from build123d import *
from build123d import SkipClean  # not in build123d's __all__

# Parameters (mm, degrees)
F0_R     = 2.775
F0_R_2   = 1.275
F1_DEPTH = 2


with BuildPart() as f1:
    # F0 (on Top) → F1 (new body)
    with BuildSketch(Plane.XY):
        with BuildLine():
            Line((0, 28.575), (-45, 28.575))
            Line((-45, 28.575), (-45, -28.575))
            Line((-45, -28.575), (0, -28.575))
            Line((0, -28.575), (0, -27.8123737215))
            ThreePointArc((0, -27.8123737215), (-2.775, -25.0373737215), (0, -22.2623737215))
            Line((0, -22.2623737215), (0, 28.575))
        make_face()
        with Locations((-39, 25.075)):
            Circle(F0_R, mode=Mode.SUBTRACT)
        with BuildLine():
            Line((0, -23.7623737215), (0, -22.2623737215))
            ThreePointArc((0, -22.2623737215), (-2.775, -25.0373737215), (0, -27.8123737215))
            Line((0, -27.8123737215), (0, -26.3123737215))
            ThreePointArc((0, -26.3123737215), (-1.275, -25.0373737215), (0, -23.7623737215))
        make_face()
        with Locations((-39, 25.075)):
            Circle(F0_R)
        with Locations((-39, 25.075)):
            Circle(F0_R_2, mode=Mode.SUBTRACT)
    extrude(amount=F1_DEPTH)

    # F2: F1 across face


with BuildPart() as f1_1:
    add(f1.part, clean=False)
    with SkipClean():  # cleaning this boolean's faces spoils the solid; the shape is the same uncleaned
        add(f1.part.mirror(Plane(origin=(0, 2.4063131393, 1), x_dir=(0, 1, 0), z_dir=(1, 0, 0))), clean=False)


solid = f1_1.part
The listing builds one solid part. Answer for the finished solid, in the listing's coordinates (mm). Coordinates: 2 decimals unless noted, no trailing zeros. Write each loop counter-clockwise with the first axis right and the second up, starting at its lowest first coordinate (ties: lowest second). Pieces come first, ordered by that corner, then holes. Notation, with made-up numbers: (61, 9) - (87, 9) arc R13 cw to (87, 22) - close; hole circle Ø3 at (66, 80). An arc over 180 degrees is marked (long way). Return JSON: item names as keys, results as strings.
1. For a pull along Y with two mould halves and no side action, classify faces 1 (the face through (1, -28.575, 1)), 2 (the face through (-45, 0, 1)), 3 (the face through (0.056, -23.764, 0.986)) as +Y half, -Y half, draft (parallel to the pull), parting line (faces both ways), or undercut.
Final values:
{"face 1": "-Y half", "face 2": "draft", "face 3": "undercut"}
2. Consider line 1 along X through (y, z) = (-25, 0.35); line 2 along Y through (x, z) = (-39, 0.65) (3 decimals); line 3 along X through (y, z) = (24.5, 0.65). Determine where each line is inside the solid, lowest interval first.
Final values:
{"line 1": "-45 to -1.27, 1.27 to 45", "line 2": "-28.575 to 23.8, 26.35 to 28.575", "line 3": "-45 to -40.14, -37.86 to 37.86, 40.14 to 45"}
3. The part is cut by section B-B on y = -25. Determine the outline of the cut face in (x, z).
Final values:
{"outline": "(-45, 0) - (-1.27, 0) - (-1.27, 2) - (-45, 2) - close; (1.27, 0) - (45, 0) - (45, 2) - (1.27, 2) - close"}
4. The part is cut by section A-A on x = 0. Determine the outline of the cut face in (y, z) (3 decimals), then the cut area to 3 significant figures.
Final values:
{"outline": "(-28.575, 0) - (-26.312, 0) - (-26.312, 2) - (-28.575, 2) - close; (-23.762, 0) - (28.575, 0) - (28.575, 2) - (-23.762, 2) - close", "area": "109 mm^2"}
